Verification items for this drawing (mm, ordinates from the low corner). Coordinates: 2 decimals unless noted, no trailing zeros. Write each loop counter-clockwise with the first axis right and the second up, starting at its lowest first coordinate (ties: lowest second). Pieces come first, ordered by that corner, then holes. Notation, with made-up numbers: M 82,43 L 91,43 A20 ccw 91,50 Z; hole C 20.5,63.25 d3. An arc over 180 degrees is marked long. Put each result on its own line as item: value. Start each with the question number.
1) Cross-section at A-A on z = 27. Record the cut outline in (x, y), plus the area to 3 significant figures.
2) Mould release check, pull along X, two halves, no side actions. Record for the marked faces 1, 2 and 3: released by +X, released by -X, zero draft, split by the parting line, or undercut.
3) Scan lines: line 1 along Y through (x, z) = (4.5, 2.5); line 2 along Y through (x, z) = (45.5, 14.5); line 3 along X through (y, z) = (6, 19). Record each from-to range of solid material in increasing order.
4) Gauge pin test, flat ends, axial feed: pin 1 (1.6 mm diameter, centred on y = 51.5, z = 10.5, fed in from -X); pin 2 (1.2 mm diameter, centred on y = 51.5, z = 10.5, fed in from +X); pin 3 (3 mm diameter, centred on y = 7, z = 19.5, fed in from +X). Record the tip position at first contact, or that the pin passes through.
5) Cross-section at B-B on x = 11.5. Record the cut outline in (y, z).
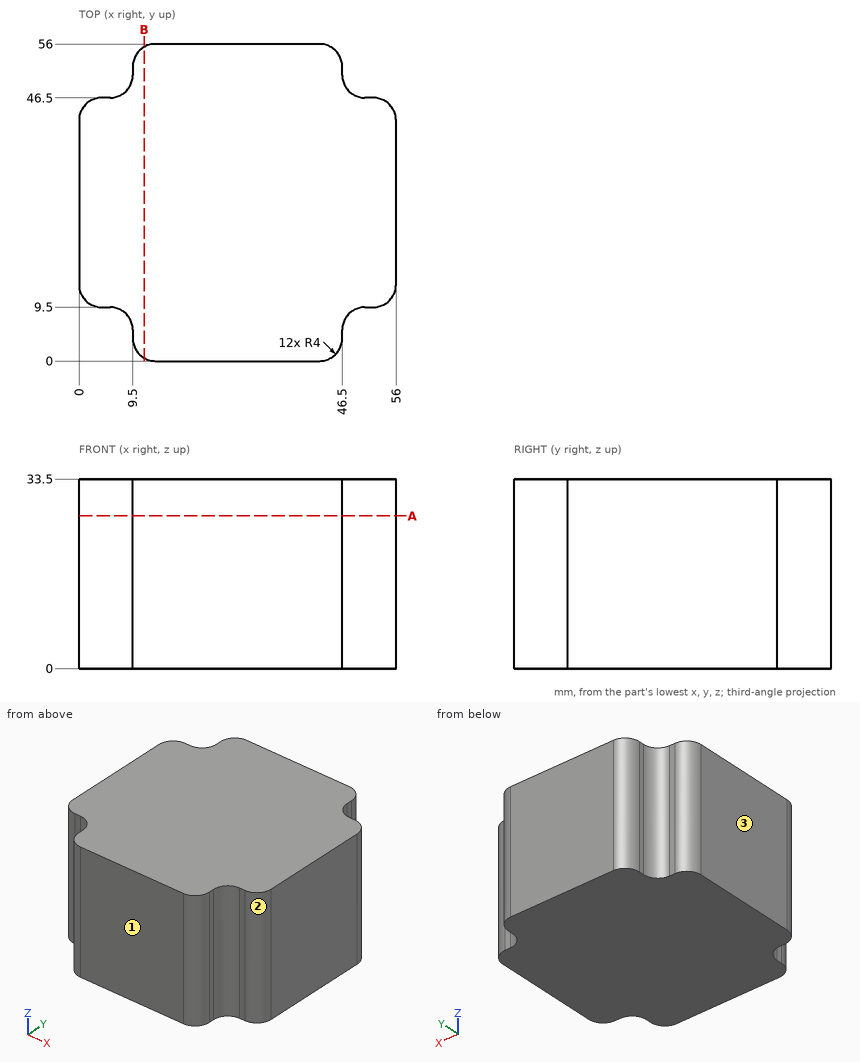
Answer key:
1. outline: M 0,13.5 A4 ccw 4,9.5 L 5.5,9.5 A4 cw 9.5,5.5 L 9.5,4 A4 ccw 13.5,0 L 42.5,0 A4 ccw 46.5,4 L 46.5,5.5 A4 cw 50.5,9.5 L 52,9.5 A4 ccw 56,13.5 L 56,42.5 A4 ccw 52,46.5 L 50.5,46.5 A4 cw 46.5,50.5 L 46.5,52 A4 ccw 42.5,56 L 13.5,56 A4 ccw 9.5,52 L 9.5,50.5 A4 cw 5.5,46.5 L 4,46.5 A4 ccw 0,42.5 Z
1. area: 2,760 mm²
2. face 1: zero draft
2. face 2: released by +X
2. face 3: released by -X
3. line 1: y = 9.5 to 46.5
3. line 2: y = 1.35 to 54.65
3. line 3: x = 9.47 to 46.53
4. pin 1: stops at x = 9.5
4. pin 2: stops at x = 46.5
4. pin 3: stops at x = 47.85
5. outline: M 0.54,0 L 55.46,0 L 55.46,33.5 L 0.54,33.5 Z
